```python
from build123d import *

# Parameters (mm, degrees)
F0_R     = 5.55625
F0_W     = 4.4338748
F0_H     = 3.3354461193
F0_W_2   = 4.4338805894
F0_H_2   = 3.1579534903
F1_DEPTH = 6.35
F2_DEPTH = 9.525


with BuildPart() as f1:
    # F0 (on Front) → F1 (new body)
    with BuildSketch(Plane.XZ):
        with BuildLine():
            ThreePointArc((2.2169431894, -8.4451103875), (6.9134438518, -5.3328248302), (8.73125, 0))
            ThreePointArc((8.73125, 0), (6.9134420239, 5.3328271999), (2.2169374, 8.4451119073))
            ThreePointArc((2.2169374, 8.4451119073), (0, 8.73125), (-2.2169374, 8.4451119073))
            ThreePointArc((-2.2169374, 8.4451119073), (-8.73125, 0), (-2.2169374, -8.4451119073))
            ThreePointArc((-2.2169374, -8.4451119073), (2.9928e-06, -8.73125), (2.2169431894, -8.4451103875))
        make_face()
        Circle(F0_R, mode=Mode.SUBTRACT)
        with BuildLine():
            ThreePointArc((-2.2169374, 8.4451119073), (0, 8.73125), (2.2169374, 8.4451119073))
            Line((2.2169374, 8.4451119073), (2.2169374, 19.2380044443))
            Line((2.2169374, 19.2380044443), (-2.2169374, 19.2380044443))
            Line((-2.2169374, 19.2380044443), (-2.2169374, 8.4451119073))
        make_face()
        with Locations((0, 20.9057275039)):
            Rectangle(F0_W, F0_H)
        with BuildLine():
            Line((-2.2169374, 22.5734505636), (2.2169374, 22.5734505636))
            Line((2.2169374, 22.5734505636), (2.2169374, 24.4680076557))
            ThreePointArc((2.2169374, 24.4680076557), (0.0079970052, 22.9441930949), (-2.2169374, 24.444558176))
            Line((-2.2169374, 24.444558176), (-2.2169374, 22.5734505636))
        make_face()
        with BuildLine():
            ThreePointArc((-2.2169374, 24.444558176), (0.0079970052, 22.9441930949), (2.2169374, 24.4680076557))
            ThreePointArc((2.2169374, 24.4680076557), (2.3363839293, 24.8893342153), (2.3766534396, 25.3254097933))
            ThreePointArc((2.3766534396, 25.3254097933), (-0.4530466345, 27.6640512993), (-2.2169374, 24.444558176))
        make_face()
        with BuildLine():
            ThreePointArc((2.38125, -26.1828773278), (2.3398127631, -25.7405790163), (2.2169431894, -25.3136739814))
            ThreePointArc((2.2169431894, -25.3136739814), (7.9302e-06, -23.8016273278), (-2.2169374, -25.3136592154))
            ThreePointArc((-2.2169374, -25.3136592154), (-0.4423061037, -28.5226886179), (2.38125, -26.1828773278))
        make_face()
        with BuildLine():
            Line((2.2169431894, -19.4155004973), (2.2169431894, -8.4451103875))
            ThreePointArc((2.2169431894, -8.4451103875), (2.9928e-06, -8.73125), (-2.2169374, -8.4451119073))
            Line((-2.2169374, -8.4451119073), (-2.2169374, -19.4155004973))
            Line((-2.2169374, -19.4155004973), (2.2169431894, -19.4155004973))
        make_face()
        with Locations((2.8947e-06, -20.9944772424)):
            Rectangle(F0_W_2, F0_H_2)
        with BuildLine():
            Line((2.2169431894, -25.3136739814), (2.2169431894, -22.5734539875))
            Line((2.2169431894, -22.5734539875), (-2.2169374, -22.5734539875))
            Line((-2.2169374, -22.5734539875), (-2.2169374, -25.3136592154))
            ThreePointArc((-2.2169374, -25.3136592154), (7.9302e-06, -23.8016273278), (2.2169431894, -25.3136739814))
        make_face()
    extrude(amount=F1_DEPTH)

    # F0 (on Front) → F2 (join)
    with BuildSketch(Plane.XZ):
        with Locations((0, 20.9057275039)):
            Rectangle(F0_W, F0_H)
        with Locations((2.8947e-06, -20.9944772424)):
            Rectangle(F0_W_2, F0_H_2)
    extrude(amount=-F2_DEPTH)


solid = f1.part
```
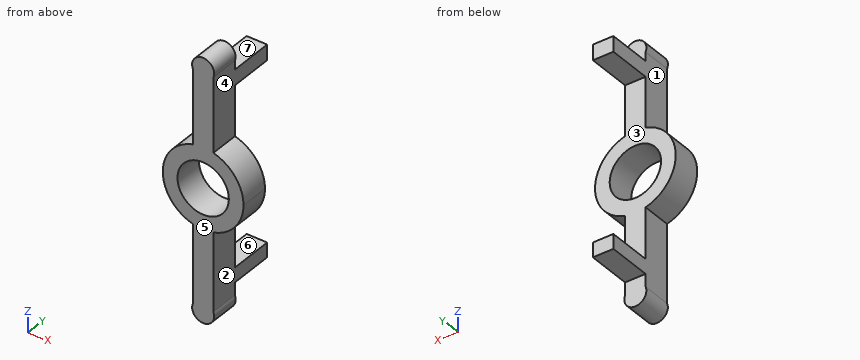
Verification items for the finished model (mm, model axes). Face numbers are marked on the shaded views. A direction names the side the tool comes from. Round coordinates to 2 decimals unless told otherwise and drop trailing zeros. Order: outer loops, then holes, each group sorted by start corner. A loop starts at its lowest first (then second) coordinate and runs counter-clockwise, first axis right, second up.
1) Cross-section at C-C, the plane z = 2.5. Record the cut outline in (x, y), plus the area to 3 significant figures.
Geometry says:
outline: (-8.37, -6.35) - (-4.96, -6.35) - (-4.96, 0) - (-8.37, 0) - close; (4.96, -6.35) - (8.37, -6.35) - (8.37, 0) - (4.96, 0) - close
area: 43.2 mm2
2) Tool access check on the marked faces 1, 2 and 3. Record the directions out of +Z, -Z, +X, -X, +Y, -Y that give a thin tool (end or side, any length) a straight path to the whole face; none if there is none.
Geometry says:
face 1: -X, +Y, -Y
face 2: +X, +Y, -Y
face 3: +X, -X, +Y
3) Draft check along Z on the marked faces 4, 5, 6 and 7. Enter one of: +Z half, -Z half, draft (parallel to the pull), parting line (faces both ways), or undercut.
Geometry says:
face 4: undercut
face 5: draft
face 6: undercut
face 7: +Z half
4) Cross-section at B-B, the plane y = -0.75. Record the cut outline in (x, z).
Geometry says:
outline: (-2.22, -25.31) arc R2.38 ccw (long way) to (2.22, -25.31) - (2.22, -8.45) arc R8.73 ccw to (2.22, 8.45) - (2.22, 24.47) arc R2.38 ccw (long way) to (-2.22, 24.44) - (-2.22, 8.45) arc R8.73 ccw to (-2.22, -8.45) - close; hole circle Ø11.11 at (0, 0)
5) Cross-section at D-D, the plane z = -15. Record the cut outline in (x, y).
Geometry says:
outline: (-2.22, -6.35) - (2.22, -6.35) - (2.22, 0) - (-2.22, 0) - close
6) Depth check by flat-ended pin: pin 1 (5 mm diameter, centred on y = 4.5, z = -20, fed in from +X); pin 2 (1.4 mm diameter, centred on x = 0.5, z = 25.5, fed in from +Y); pin 3 (3 mm diameter, centred on x = -0.5, y = 4.5, fed in from +Z); pin 4 (4 mm diameter, centred on x = -1.5, y = 1, fed in from +Z). Enter the tip coordinate at first touch or a pass-through.
Geometry says:
pin 1: stops at x = 2.22
pin 2: stops at y = 0
pin 3: stops at z = 22.57
pin 4: stops at z = 27.71
7) Material ranges on line 1 (Z direction, x = 0, y = -5); line 2 (Z direction, x = 1.5, y = 3.75); line 3 (X direction, y = -1, z = 14), recorded low to high.
Geometry says:
line 1: z = -28.56 to -5.56, 5.56 to 27.71
line 2: z = -22.57 to -19.42, 19.24 to 22.57
line 3: x = -2.22 to 2.22
